Source: CAD feature listing. Evaluate the final solid. Frame: model axes, mm. Face numbers are marked on the shaded views. Give positions to 0.01 mm unless a question says otherwise; leave off trailing zeros. Write each loop counter-clockwise with the first axis right and the second up, starting at its lowest first coordinate (ties: lowest second). Pieces come first, ordered by that corner, then holes. Notation, with made-up numbers: (2, 22.5) - (52, 22.5) arc R18 ccw to (52, 45.5) - close; hole circle Ø2 at (45, -36). An arc over 180 degrees is marked (long way). One line per question, with ' | ' between items. Start each with the question number.
(1) Pin query (flat end, axial travel): pin 1 (4 mm diameter, centred on x = -1.5, y = 0, fed in from +Z). Return the tip coordinate at first contact, or that it passes through.
(2) Ray query, line 1 (Y direction, x = 1.5, z = 1.45); line 2 (X direction, y = -1, z = 1.7) (3 decimals); line 3 (Z direction, x = -2, y = -3.75). Return the intervals inside material, ascending. Write a range as [from, to].
(3) Section A-A, the plane z = 1.55. Return loops of the section in (x, y) (3 decimals), plus the area to 3 significant figures.
(4) Draft query along Y for the marked faces 1 and 2. Return one class per face: +Y half, -Y half, draft (parallel to the pull), parting line (faces both ways), or undercut.
(5) Section B-B, the plane y = 1.5. Return loops of the section in (x, z) (3 decimals), plus the area to 3 significant figures.
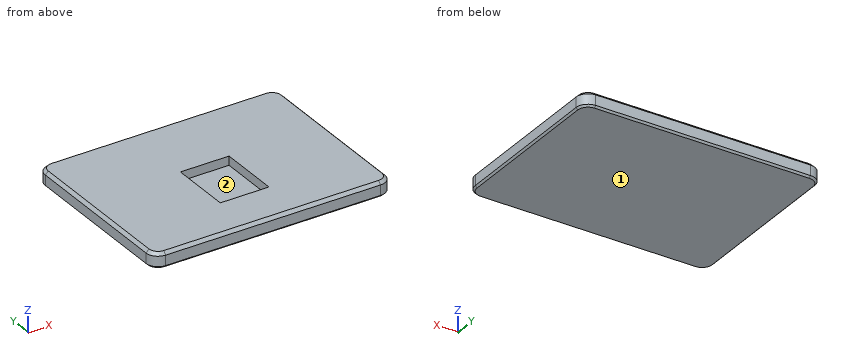
```python
from build123d import *

# Parameters (mm, degrees)
SKETCH1_W           = 40
SKETCH1_H           = 30
BOSS_EXTRUDE1_DEPTH = 2.5
SKETCH2_W           = 8.15
SKETCH2_H           = 10.3
CUT_EXTRUDE1_DEPTH  = 1.5
FILLET1_R           = 2
CHAMFER1_SIZE       = 0.5
CHAMFER2_SIZE       = 0.3


with BuildPart() as part:
    # Sketch1 → Boss-Extrude1 (new body)
    with BuildSketch(Plane.XY):
        Rectangle(SKETCH1_W, SKETCH1_H)
    extrude(amount=BOSS_EXTRUDE1_DEPTH)

    # Sketch2 → Cut-Extrude1 (cut)
    with BuildSketch(Plane.XY.offset(2.5)):
        with Locations((0, -2.5)):
            Rectangle(SKETCH2_W, SKETCH2_H)
    extrude(amount=-CUT_EXTRUDE1_DEPTH, mode=Mode.SUBTRACT)

    # Fillet1
    fillet1_edges = [part.edges().sort_by_distance(p)[0] for p in [
        (20, -15, 1.25),
        (-20, -15, 1.25),
        (-20, 15, 1.25),
        (20, 15, 1.25),
    ]]
    fillet(fillet1_edges, radius=FILLET1_R)

    # Chamfer1
    chamfer1_edges = [part.edges().sort_by_distance(p)[0] for p in [
        (0, -15, 2.5),
        (-20, 0, 2.5),
        (20, 0, 2.5),
        (0, 15, 2.5),
        (19.414213562, 14.414213562, 2.5),
        (-19.414213562, 14.414213562, 2.5),
        (19.414213562, -14.414213562, 2.5),
        (-19.414213562, -14.414213562, 2.5),
    ]]
    chamfer(chamfer1_edges, length=CHAMFER1_SIZE)

    # Chamfer2
    chamfer2_edges = [part.edges().sort_by_distance(p)[0] for p in [
        (0, -15, 0),
        (20, 0, 0),
        (-20, 0, 0),
        (0, 15, 0),
        (19.414213562, 14.414213562, 0),
        (-19.414213562, 14.414213562, 0),
        (19.414213562, -14.414213562, 0),
        (-19.414213562, -14.414213562, 0),
    ]]
    chamfer(chamfer2_edges, length=CHAMFER2_SIZE)


solid = part.part
```
Check sheet entries:
1) pin 1: z = 1
2) line 1: [-15, -7.65], [2.65, 15] | line 2: [-20, -4.075], [4.075, 20] | line 3: [0, 1]
3) outline: (-20, -13) arc R2 ccw to (-18, -15) - (18, -15) arc R2 ccw to (20, -13) - (20, 13) arc R2 ccw to (18, 15) - (-18, 15) arc R2 ccw to (-20, 13) - close; hole (-4.075, -7.65) - (4.075, -7.65) - (4.075, 2.65) - (-4.075, 2.65) - close | area: 1,110 mm²
4) face 1: draft | face 2: undercut
5) outline: (-20, 0.3) - (-19.7, 0) - (19.7, 0) - (20, 0.3) - (20, 2) - (19.5, 2.5) - (4.075, 2.5) - (4.075, 1) - (-4.075, 1) - (-4.075, 2.5) - (-19.5, 2.5) - (-20, 2) - close | area: 87.4 mm²
